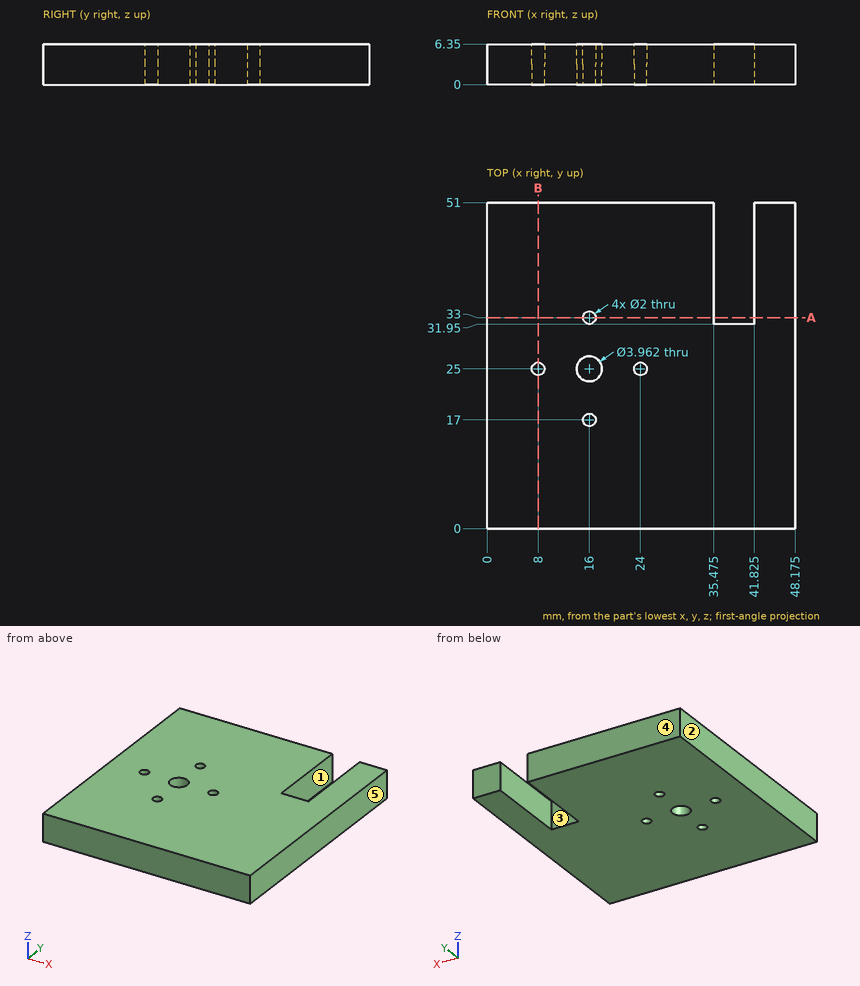
Source: three-view drawing plus pictorial views. Frame: mm from the lowest corner of the part. A direction names the side the tool comes from. Round coordinates to 2 decimals unless told otherwise and drop trailing zeros. Loops run counter-clockwise (first coordinate to the right, second up) from the corner with the lowest first, then second, coordinate; pieces in that order, holes last. Notation, with made-up numbers: M 39,-2 L 46,-2 A17 ccw 46,5 Z; hole C 18.5,62 d3. An arc over 180 degrees is marked long. Put each result on its own line as item: value.
(1) Access query for the marked faces 1 and 2. Directions: +Z, -Z, +X, -X, +Y, -Y. A direction counts if a zero-diameter tool reaches every point of the face in a straight line with its end or side. Return the directions, or none.
Solutions:
face 1: +Z, -Z, +Y
face 2: +Z, -Z, -X, +Y, -Y
(2) Section A-A, the plane y = 33. State how many separate pieces and enclosed holes the cut face has, and give its area (3 significant figures).
Solutions:
separate pieces: 3
enclosed holes: 0
area: 253 mm²
(3) Ray query, line 1 (X direction, y = 25, z = 4.35) (1 decimal); line 2 (Y direction, x = 16, z = 5.6); line 3 (Y direction, x = 24, z = 2.75). Return the intervals inside material, ascending. Write a range as [from, to].
Solutions:
line 1: [0, 7], [9, 14], [18, 23], [25, 48.2]
line 2: [0, 16], [18, 23.02], [26.98, 32], [34, 51]
line 3: [0, 24], [26, 51]
(4) Section B-B, the plane x = 8. Return loops of the section in (y, z).
Solutions:
outline: M 0,0 L 24,0 L 24,6.35 L 0,6.35 Z; M 26,0 L 51,0 L 51,6.35 L 26,6.35 Z
(5) Pull-direction query (X, two-part tool) for the marked faces 3, 4 and 5; classes: released by +X, released by -X, zero draft, split by the parting line, or undercut.
Solutions:
face 3: undercut
face 4: zero draft
face 5: released by +X
(6) First-contact query: pin 1 (2 mm diameter, centred on x = 39, z = 3.5, fed in from +Y). Flat tip, straight axial feed; report the tip coordinate or a pass-through.
Solutions:
pin 1: y = 31.95
